Work out the finished part from the listing and answer in its coordinate system (mm). Face numbers are marked on the shaded views. A direction names the side the tool comes from. Give positions to 0.01 mm unless a question says otherwise; leave off trailing zeros. Order: outer loops, then holes, each group sorted by start corner. A loop starts at its lowest first (then second) coordinate and runs counter-clockwise, first axis right, second up. Notation, with made-up numbers: M 75.5,-31.75 L 125.5,-31.75 A14 cw 125.5,-17.75 Z; hole C -15,25 d5. An arc over 180 degrees is marked long. One line per item, written item: value.
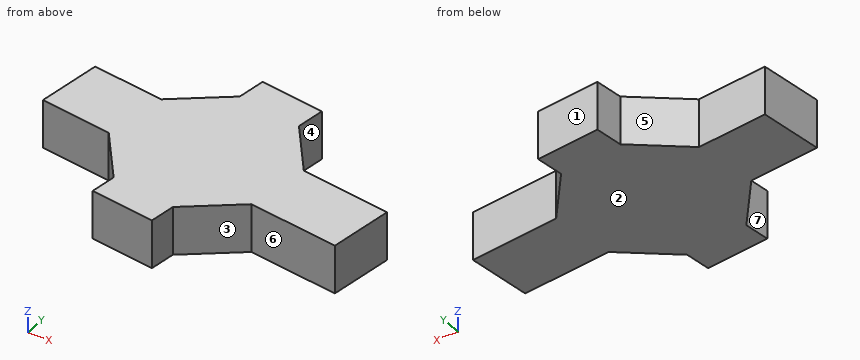
from build123d import *

# Parameters (mm, degrees)
F1_DEPTH = 37.1
F2_DEPTH = 56.1
F3_DEPTH = 71
F4_DEPTH = 20.3
F5_DEPTH = 22.2


with BuildPart() as f1:
    # F0 (on Top) → F1 (new body)
    with BuildSketch(Plane.XY):
        Polygon((-56.8497114772, 33.5975717617), (-63.9558873182, -16.4417456699), (-33.5975717617, -56.8497114772), (16.4417456699, -63.9558873182), (56.8497114772, -33.5975717617), (63.9558873182, 16.4417456699), (33.5975717617, 56.8497114772), (-16.4417456699, 63.9558873182), align=None)
    extrude(amount=F1_DEPTH)

    # F2 (add): a face of the model
    f2_faces = [f1.faces().sort_by_distance(p)[0] for p in [
        (-60.4027993977, 8.5779130459, 18.55),
    ]]
    extrude(f2_faces, amount=F2_DEPTH)

    # F3 (add): a face of the model
    f3_faces = [f1.faces().sort_by_distance(p)[0] for p in [
        (60.4027993977, -8.5779130459, 18.55),
    ]]
    extrude(f3_faces, amount=F3_DEPTH)

    # F4 (add): a face of the model
    f4_faces = [f1.faces().sort_by_distance(p)[0] for p in [
        (-8.5779130459, -60.4027993977, 18.55),
    ]]
    extrude(f4_faces, amount=F4_DEPTH)

    # F5 (add): a face of the model
    f5_faces = [f1.faces().sort_by_distance(p)[0] for p in [
        (8.5779130459, 60.4027993977, 18.55),
    ]]
    extrude(f5_faces, amount=F5_DEPTH)


solid = f1.part
(1) Find the intervals of material crossed by probe 1 along X at (y, z) = (24, 24.5); probe 2 along Y at (x, z) = (-80.5, 17); probe 3 along X at (y, z) = (-4, 32.5), in increasing order. Write a range as from..to.
Findings:
probe 1: x = -114.88..58.28
probe 2: y = -14.09..36.96
probe 3: x = -118.85..132.77
(2) Section D-D, the plane y = -23 is taken. Give the vertices of the cut face in (x, z).
Findings:
outline: M -59.03,0 L 130.07,0 L 130.07,37.1 L -59.03,37.1 Z
(3) Determine the mould class of the marked faces 1, 2 and 3 for opening direction X: pulls with the +X half, pulls with the -X half, needs draft (parallel to the pull), parting line crosses it, or undercut.
Findings:
face 1: pulls with the +X half
face 2: needs draft
face 3: undercut
(4) Section B-B, the plane z = 15 is taken. Give the vertices of the cut face in (x, y), then the cut area to 3 significant figures.
Findings:
outline: M -119.5,-8.55 L -63.96,-16.44 L -33.6,-56.85 L -36.45,-76.95 L 13.59,-84.05 L 16.44,-63.96 L 56.85,-33.6 L 127.14,-43.58 L 134.25,6.46 L 63.96,16.44 L 33.6,56.85 L 36.72,78.83 L -13.32,85.94 L -16.44,63.96 L -56.85,33.6 L -112.39,41.49 Z
area: 20,900 mm^2
(5) Section C-C, the plane x = 68.5 is taken. Give the vertices of the cut face in (y, z), then the cut area to 3 significant figures.
Findings:
outline: M -35.25,0 L 15.8,0 L 15.8,37.1 L -35.25,37.1 Z
area: 1,890 mm^2
(6) Which of the six approach directions +Z, -Z, +X, -X, +Y, -Y give full straight-line access (tool end or side, diameter ignored) to the marked faces 4, 5, 6 and 7?
Findings:
face 4: +Z, -Z, +X
face 5: +Z, -Z, +Y
face 6: +Z, -Z, -Y
face 7: +Z, -Z, -X
(7) Section A-A, the plane y = -40.5 is taken. Give the vertices of the cut face in (x, z).
Findings:
outline: M -45.88,0 L 47.66,0 L 47.66,37.1 L -45.88,37.1 Z; M 105.45,0 L 127.58,0 L 127.58,37.1 L 105.45,37.1 Z
(8) Given P1, Ø1.5, axis at x = -63.5, z = 5.5, coming from the +Y side; P2, Ø4, axis at x = -84.5, z = 28, coming from the -Y side; P3, Ø6, axis at x = -55, z = 17.5, coming from the -Y side, each flat-ended and moving along its own axis, determine where each tip first touches the part or whether it passes through.
Findings:
P1: stops at y = 34.65
P2: stops at y = -13.81
P3: stops at y = -32.36
